Verification items for this drawing (mm, ordinates from the low corner). Coordinates: 2 decimals unless noted, no trailing zeros. Write each loop counter-clockwise with the first axis right and the second up, starting at its lowest first coordinate (ties: lowest second). Pieces come first, ordered by that corner, then holes. Notation, with made-up numbers: M -25,6 L 27,6 A17 cw 27,30 Z; hole C -26.75,46.25 d7. An arc over 180 degrees is marked long. Put each result on its own line as item: value. Start each with the question number.
1) Mould release check, pull along Z, two halves, no side actions. Record for the marked faces 1 and 2: released by +Z, released by -Z, zero draft, split by the parting line, or undercut.
2) Gauge pin test, flat ends, axial feed: pin 1 (1.9 mm diameter, centred on x = 169, y = 2, fed in from -Z); pin 2 (20.5 mm diameter, centred on x = 241.3, z = 88.9, fed in from -Y); pin 3 (11.5 mm diameter, centred on x = 63.5, z = 88.9, fed in from -Y). Record the tip position at first contact, or that the pin passes through.
3) Cross-section at B-B on x = 63.5. Record the cut outline in (y, z).
4) Scan lines: line 1 along X through (y, z) = (4.9, 50.8) (1 decimal); line 2 along X through (y, z) = (5.1, 88.9); line 3 along X through (y, z) = (2.75, 153). Record each from-to range of solid material in increasing order.
5) Cross-section at A-A on z = 156.5. Record the cut outline in (x, y).
6) Cross-section at C-C on x = 152.4. Count the separate pieces of the cut face and the enclosed holes in it, plus the area to 3 significant figures.
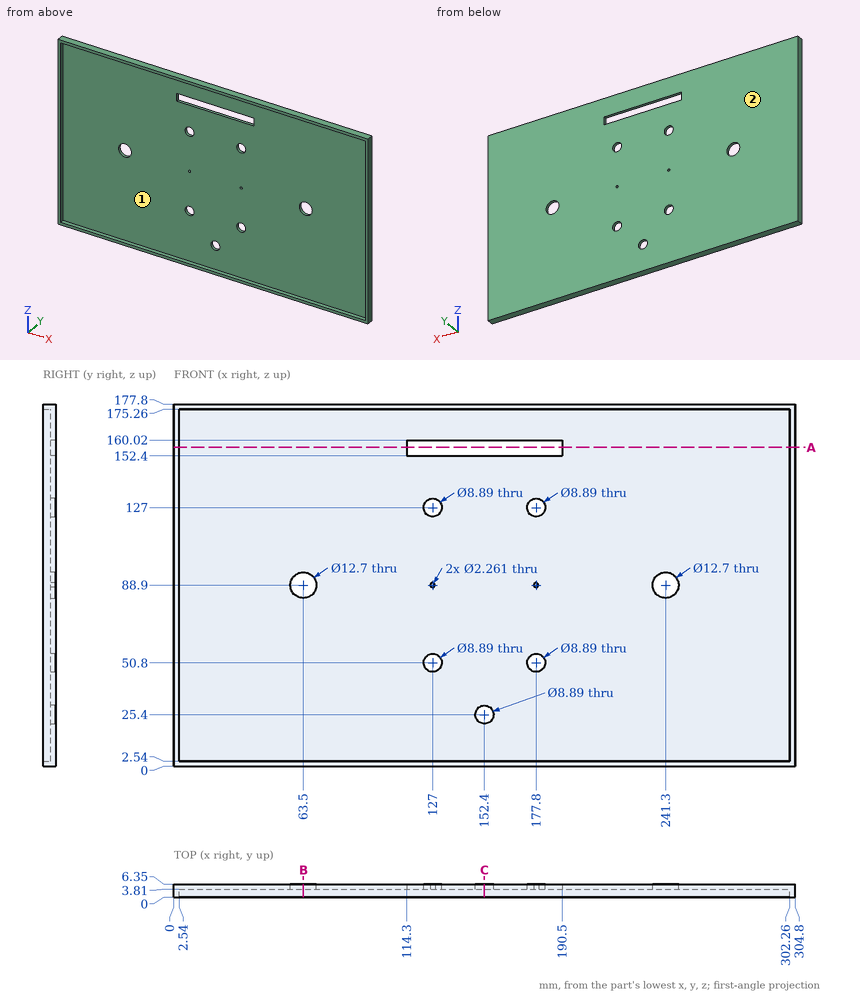
Answer key:
1. face 1: undercut
1. face 2: zero draft
2. pin 1: stops at z = 0
2. pin 2: stops at y = 3.81
2. pin 3: passes through
3. outline: M 0,0 L 6.35,0 L 6.35,82.55 L 3.81,82.55 L 3.81,2.54 L 0,2.54 Z; M 0,175.26 L 3.81,175.26 L 3.81,95.25 L 6.35,95.25 L 6.35,177.8 L 0,177.8 Z
4. line 1: x = 0 to 122.6, 131.4 to 173.4, 182.2 to 304.8
4. line 2: x = 0 to 57.15, 69.85 to 125.87, 128.13 to 176.67, 178.93 to 234.95, 247.65 to 304.8
4. line 3: x = 0 to 2.54, 302.26 to 304.8
5. outline: M 0,0 L 2.54,0 L 2.54,3.81 L 114.3,3.81 L 114.3,6.35 L 0,6.35 Z; M 190.5,3.81 L 302.26,3.81 L 302.26,0 L 304.8,0 L 304.8,6.35 L 190.5,6.35 Z
6. separate pieces: 3
6. enclosed holes: 0
6. area: 429 mm²
